Geometry check sheet. Reference: the model listing, model coordinates, mm. A direction names the side the tool comes from. Round coordinates to 2 decimals unless told otherwise and drop trailing zeros. Loops run counter-clockwise (first coordinate to the right, second up) from the corner with the lowest first, then second, coordinate; pieces in that order, holes last. Notation, with made-up numbers: (0, 6) - (41, 6) arc R25 cw to (41, 20) - close; hole circle Ø6 at (-7.5, -40). An arc over 180 degrees is marked (long way). Answer as CSV lines item,"result". Start each with the question number.
1) Access from +Z, -Z, +X, -X, +Y, -Y to the whole of each face (thin tool, end or side, straight path). Record for faces 1 (the flat face through (31.21, -41.25, 15.65)), 2 (the flat face through (-29, 28.229, 24)), 3 (the flat face through (-29, 0, 12.7)).
2) Cross-section at A-A on y = 24.8. Record the boundary of the cut face in (x, z), and give its area (3 significant figures).
3) Draft check along Y on faces 4 (the flat face through (0, -42.5, 16)), 5 (the cylindrical face through (23.113, 31.965, 5.596)), 6 (the flat face through (32.5, -1, 16)). Enter one of: released by +Y, released by -Y, zero draft, split by the parting line, or undercut.
4) Cross-section at C-C on x = -13.5. Record the boundary of the cut face in (y, z).
5) Depth check by flat-ended pin: P1, Ø2, axis at x = 23, y = 31.5, coming from the +Z side; P2, Ø1.1, axis at x = -29.365, y = -39.365, coming from the +Z side; P3, Ø6, axis at x = 5.5, y = -4, coming from the +Z side; P4, Ø1.6, axis at x = 22.225, y = 32.004, coming from the -Z side. Enter the tip coordinate at first touch or a pass-through.
6) Cross-section at B-B on z = 27. Record the boundary of the cut face in (x, y) (3 decimals).
7) Thickness scan on line 1 along X through (y, z) = (32, 6.5); line 2 along X through (y, z) = (12.5, 11); line 3 along Y through (x, z) = (19.5, 17). Record the ranges inside material, lowest first.
8) Cross-section at D-D on z = 15.5. Record the boundary of the cut face in (x, y) (3 decimals).
from build123d import *

# Parameters (mm, degrees)
SKETCH1_W           = 55
SKETCH1_H           = 75
SKETCH1_R           = 0.889
BOSS_EXTRUDE1_DEPTH = 5
SKETCH2_W           = 65
SKETCH2_H           = 85
SKETCH2_W_2         = 55
SKETCH2_H_2         = 75
BOSS_EXTRUDE2_DEPTH = 31.75
CUT_EXTRUDE1_REACH  = 85.901
SKETCH4_R           = 5.207
CUT_EXTRUDE2_DEPTH  = 2.46
CHAMFER1_SIZE       = 2.54
SKETCH5_R           = 0.889
CUT_EXTRUDE3_DEPTH  = 19.05
SKETCH6_R           = 3.429
SKETCH6_R_2         = 0.889
BOSS_EXTRUDE3_DEPTH = 6.35


with BuildPart() as part:
    # Sketch1 → Boss-Extrude1 (new body)
    with BuildSketch(Plane.XY):
        Rectangle(SKETCH1_W, SKETCH1_H)
        with Locations((-22.225, 32.004)):
            Circle(SKETCH1_R, mode=Mode.SUBTRACT)
        with Locations(Location((-22.225, -32.004, 0), (0, 0, 180))):
            Circle(SKETCH1_R, mode=Mode.SUBTRACT)
        with Locations((22.225, -32.004)):
            Circle(SKETCH1_R, mode=Mode.SUBTRACT)
        with Locations(Location((22.225, 32.004, 0), (0, 0, 180))):
            Circle(SKETCH1_R, mode=Mode.SUBTRACT)
    extrude(amount=BOSS_EXTRUDE1_DEPTH)

    # Sketch2 → Boss-Extrude2 (add)
    with BuildSketch(Plane(origin=(0, 0, 0), x_dir=(-1, 0, 0), z_dir=(0, 0, -1))):
        Rectangle(SKETCH2_W, SKETCH2_H)
        Rectangle(SKETCH2_W_2, SKETCH2_H_2, mode=Mode.SUBTRACT)
    extrude(amount=-BOSS_EXTRUDE2_DEPTH)

    # Sketch3 → Cut-Extrude1 (cut, up to next)
    with BuildSketch(Plane.ZY.offset(32.5), mode=Mode.PRIVATE) as cut_extrude1_sk1:
        with BuildLine():
            Line((25.868155142, 21.371), (22.264844858, 21.371))
            ThreePointArc((22.264844858, 21.371), (20.193, 24.8), (22.264844858, 28.229))
            Line((22.264844858, 28.229), (25.868155142, 28.229))
            ThreePointArc((25.868155142, 28.229), (27.94, 24.8), (25.868155142, 21.371))
        make_face()
    cut_extrude1_tool1 = extrude(cut_extrude1_sk1.sketch, amount=-CUT_EXTRUDE1_REACH, mode=Mode.PRIVATE) & part.part
    add(cut_extrude1_tool1.solids().sort_by_distance((-32.5, 24.8, 24.0665))[0], mode=Mode.SUBTRACT)

    # Sketch4 → Cut-Extrude2 (cut)
    with BuildSketch(Plane.ZY.offset(32.5)):
        with Locations((24.0665, 24.8)):
            Circle(SKETCH4_R)
    extrude(amount=-CUT_EXTRUDE2_DEPTH, mode=Mode.SUBTRACT)

    # Chamfer1
    chamfer1_edges = [part.edges().sort_by_distance(p)[0] for p in [
        (32.5, 42.5, 15.875),
        (-32.5, 42.5, 15.875),
        (-32.5, -42.5, 15.875),
        (32.5, -42.5, 15.875),
    ]]
    chamfer(chamfer1_edges, length=CHAMFER1_SIZE)

    # Sketch5 → Cut-Extrude3 (cut)
    with BuildSketch(Plane.XY.offset(31.75)):
        with Locations((29.365, 39.365)):
            Circle(SKETCH5_R)
        with Locations((29.365, -39.365)):
            Circle(SKETCH5_R)
        with Locations((-29.365, -39.365)):
            Circle(SKETCH5_R)
        with Locations((-29.365, 39.365)):
            Circle(SKETCH5_R)
        with Locations((29.365, 0)):
            Circle(SKETCH5_R)
        with Locations((-29.365, 0)):
            Circle(SKETCH5_R)
    extrude(amount=-CUT_EXTRUDE3_DEPTH, mode=Mode.SUBTRACT)

    # Sketch6 → Boss-Extrude3 (add)
    # profile 1 of 4: a face of its own
    with BuildSketch(Plane.XY.offset(5)):
        with Locations(Location((-22.225, 32.004, 0), (0, 0, 180))):
            Circle(SKETCH6_R)
        with Locations((-22.225, 32.004)):
            Circle(SKETCH6_R_2, mode=Mode.SUBTRACT)
    # profile 2 of 4: a face of its own
    with BuildSketch(Plane.XY.offset(5)):
        with Locations(Location((-22.225, -32.004, 0), (0, 0, 180))):
            Circle(SKETCH6_R)
        with Locations(Location((-22.225, -32.004, 0), (0, 0, 180))):
            Circle(SKETCH6_R_2, mode=Mode.SUBTRACT)
    # profile 3 of 4: a face of its own
    with BuildSketch(Plane.XY.offset(5)):
        with Locations(Location((22.225, -32.004, 0), (0, 0, 180))):
            Circle(SKETCH6_R)
        with Locations((22.225, -32.004)):
            Circle(SKETCH6_R_2, mode=Mode.SUBTRACT)
    # profile 4 of 4: a face of its own
    with BuildSketch(Plane.XY.offset(5)):
        with Locations(Location((22.225, 32.004, 0), (0, 0, 180))):
            Circle(SKETCH6_R)
        with Locations(Location((22.225, 32.004, 0), (0, 0, 180))):
            Circle(SKETCH6_R_2, mode=Mode.SUBTRACT)
    extrude(amount=BOSS_EXTRUDE3_DEPTH)


solid = part.part
Answer block:
1,face 1,"+Z, -Z, +X, -Y"
1,face 2,"-X"
1,face 3,"+Z"
2,outline,"(-32.5, 0) - (32.5, 0) - (32.5, 31.75) - (27.5, 31.75) - (27.5, 5) - (-27.5, 5) - (-27.5, 20.19) - (-30.04, 20.19) - (-30.04, 18.86) - (-32.5, 18.86) - close; (-32.5, 29.27) - (-30.04, 29.27) - (-30.04, 27.94) - (-27.5, 27.94) - (-27.5, 31.75) - (-32.5, 31.75) - close"
2,area,"547 mm^2"
3,face 4,"released by -Y"
3,face 5,"undercut"
3,face 6,"zero draft"
4,outline,"(-42.5, 0) - (42.5, 0) - (42.5, 31.75) - (37.5, 31.75) - (37.5, 5) - (-37.5, 5) - (-37.5, 31.75) - (-42.5, 31.75) - close"
5,P1,"stops at z = 11.35"
5,P2,"stops at z = 12.7"
5,P3,"stops at z = 5"
5,P4,"passes through"
6,outline,"(-32.5, -39.96) - (-29.96, -42.5) - (29.96, -42.5) - (32.5, -39.96) - (32.5, 39.96) - (29.96, 42.5) - (-29.96, 42.5) - (-32.5, 39.96) - (-32.5, 29.102) - (-30.04, 29.102) - (-30.04, 27.33) - (-27.5, 27.33) - (-27.5, 37.5) - (27.5, 37.5) - (27.5, -37.5) - (-27.5, -37.5) - (-27.5, 22.27) - (-30.04, 22.27) - (-30.04, 20.498) - (-32.5, 20.498) - close; hole circle Ø1.778 at (-29.365, -39.365); hole circle Ø1.778 at (-29.365, 0); hole circle Ø1.778 at (-29.365, 39.365); hole circle Ø1.778 at (29.365, -39.365); hole circle Ø1.778 at (29.365, 0); hole circle Ø1.778 at (29.365, 39.365)"
7,line 1,"x = -32.5 to -27.5, -25.65 to -23.11, -21.34 to -18.8, 18.8 to 21.34, 23.11 to 25.65, 27.5 to 32.5"
7,line 2,"x = -32.5 to -27.5, 27.5 to 32.5"
7,line 3,"y = -42.5 to -37.5, 37.5 to 42.5"
8,outline,"(-32.5, -39.96) - (-29.96, -42.5) - (29.96, -42.5) - (32.5, -39.96) - (32.5, 39.96) - (29.96, 42.5) - (-29.96, 42.5) - (-32.5, 39.96) - close; hole circle Ø1.778 at (-29.365, -39.365); hole circle Ø1.778 at (-29.365, 0); hole circle Ø1.778 at (-29.365, 39.365); hole (-27.5, -37.5) - (27.5, -37.5) - (27.5, 37.5) - (-27.5, 37.5) - close; hole circle Ø1.778 at (29.365, -39.365); hole circle Ø1.778 at (29.365, 0); hole circle Ø1.778 at (29.365, 39.365)"
